Can you work these out from the model? Positions are in its coordinate system, mm. A direction names the side the tool comes from. Give positions to 0.01 mm unless a question says otherwise; leave off trailing zeros. Order: outer loops, then holes, each group sorted by start corner. A loop starts at its lowest first (then second) coordinate and runs counter-clockwise, first axis right, second up. Notation, with made-up numbers: M -16.5,6.25 L 29.5,6.25 A38 cw 29.5,44.25 Z; hole C -35.75,-7.75 d8. An arc over 180 degrees is marked long. One line per question, with ' | ' between items. Start each with the question number.
1) I'm going to push flat-ended pins straight in: pin 1 Ø1.3 at (y, z) = (-0.5, 2) entering from +X; pin 2 Ø1.5 at (x, z) = (0.5, 3.5) entering from +Y; pin 3 Ø1 at (y, z) = (0.5, 2) entering from -X. Where does each tip first touch, or does it pass through?
2) If we section it at C-C, the plane y = 0: Please give me the cut outline in (x, z) (3 decimals).
3) Please list where these lines run through material, in increasing order: line 1 along Y through (x, z) = (0, 1.3); line 2 along Y through (x, z) = (0, 3.2); line 3 along Z through (x, y) = (2.2, -1.45). Write a range as [from, to].
4) If we section it at A-A, the plane z = 1: Please give me the cut outline in (x, y).
5) If we section it at B-B, the plane z = -3: Please give me the cut outline in (x, y).
6) Thinking about a two-plate mould opening in Z: for faces 4 (the flat face through (0, -2.5, -0.5)), 5 (the flat face through (0.25, 0.7, 2.6)), 6 (the flat face through (0.23, 2.64, 0)), which applies, +Z half, -Z half, draft (parallel to the pull), parting line (faces both ways), or undercut?
7) If we section it at D-D, the plane x = -1.1: Please give me the cut outline in (y, z) (3 decimals).
8) For faces 1 (the flat face through (0, 0, 0)), 2 (the cylindrical face through (-0.54, -2.44, 2.51)), 3 (the cylindrical face through (-0.106, 2.923, -0.493)), which set-ups out of +Z, -Z, +X, -X, +Y, -Y let a thin tool reach every point of the face, with its end or its side?
```python
from build123d import *

# Parameters (mm, degrees)
SKETCH1_R           = 2.5
SKETCH1_R_2         = 2
BOSS_EXTRUDE1_DEPTH = 5.1
REVOLVE1_ANGLE      = 180
SKETCH5_R           = 2.925
BOSS_EXTRUDE2_DEPTH = 1
BOSS_EXTRUDE3_DEPTH = 0.25
SKETCH13_W          = 0.5
SKETCH13_H          = 0.5
BOSS_EXTRUDE4_DEPTH = 5
CUT_EXTRUDE2_DEPTH  = 5


with BuildPart() as part:
    # Sketch1 → Boss-Extrude1 (new body)
    with BuildSketch(Plane.XY):
        Circle(SKETCH1_R)
        Circle(SKETCH1_R_2, mode=Mode.SUBTRACT)
    extrude(amount=BOSS_EXTRUDE1_DEPTH)

    # Sketch4 → Revolve1 (revolve)
    with BuildSketch(Plane.XY.offset(5.1)):
        with BuildLine():
            Line((-2, 0), (-2.5, 0))
            ThreePointArc((-2.5, 0), (0, 2.5), (2.5, 0))
            Line((2.5, 0), (2, 0))
            ThreePointArc((2, 0), (0, 2), (-2, 0))
        make_face()
    revolve(axis=Axis((-2.5, 0, 5.1), (1, 0, 0)), revolution_arc=REVOLVE1_ANGLE)

    # Sketch5 → Boss-Extrude2 (add)
    with BuildSketch(Plane(origin=(0, 0, 0), x_dir=(-1, 0, 0), z_dir=(0, 0, -1))):
        Circle(SKETCH5_R)
    extrude(amount=BOSS_EXTRUDE2_DEPTH)

    # Sketch8 → Boss-Extrude3 (add, symmetric)
    with BuildSketch(Plane(origin=(0, 0, 0), x_dir=(0, 0, -1), z_dir=(1, 0, 0))):
        Polygon((0, 1.072701591), (-3.556166294, 1.072701591), (-3.556166294, -0.218813925), (-2.37503672, 0.509733289), (-2.37503672, 0.763620955), (0, 0.763620955), align=None)
        Polygon((-3.556166294, -0.41750862), (-3.330966178, -0.41750862), (-3.330966178, -0.31503842), (-2.37503672, 0.3), (-2.37503672, -0.41750862), (0, -0.41750862), (0, -0.914245357), (-3.556166294, -0.914245357), align=None)
    extrude(amount=BOSS_EXTRUDE3_DEPTH, both=True)

    # Sketch13 → Boss-Extrude4 (add)
    with BuildSketch(Plane(origin=(0, 0, -1), x_dir=(-1, 0, 0), z_dir=(0, 0, -1))):
        with Locations((0.093693205, -1.27)):
            Rectangle(SKETCH13_W, SKETCH13_H)
        with Locations((0.093693205, 1.27)):
            Rectangle(SKETCH13_W, SKETCH13_H)
    extrude(amount=BOSS_EXTRUDE4_DEPTH)

    # Sketch14 → Cut-Extrude2 (cut)
    with BuildSketch(Plane.XY):
        with BuildLine():
            Line((1.518428464, -2.5), (-1.518428464, -2.5))
            ThreePointArc((-1.518428464, -2.5), (0, -2.925), (1.518428464, -2.5))
        make_face()
    extrude(amount=-CUT_EXTRUDE2_DEPTH, mode=Mode.SUBTRACT)


solid = part.part
```
Results found:
1) pin 1: stops at x = 2.5 | pin 2: stops at y = 2.5 | pin 3: stops at x = -2.5
2) outline: M -2.925,-1 L 2.925,-1 L 2.925,0 L 2.5,0 L 2.5,5.1 A2.5 ccw -2.5,5.1 L -2.5,0 L -2.925,0 Z; M -0.25,2.375 L 0.25,2.375 L 0.25,2.841 L -0.25,2.841 Z; M -0.25,3.201 L 0.25,3.201 L 0.25,3.556 L -0.25,3.556 Z; hole M -2,0 L 2,0 L 2,5.1 A2 ccw -2,5.1 Z
3) line 1: y = [-2.5, -2], [-0.91, -0.42], [0.76, 1.07], [2, 2.5] | line 2: y = [-2.5, -2], [-0.91, -0.23], [0, 1.07], [2, 2.5] | line 3: z = [-1, 0]
4) outline: C 0,0 d5; M -0.25,-0.91 L 0.25,-0.91 L 0.25,-0.42 L -0.25,-0.42 Z; M -0.25,0.76 L 0.25,0.76 L 0.25,1.07 L -0.25,1.07 Z; hole C 0,0 d4
5) outline: M -0.34,-1.52 L 0.16,-1.52 L 0.16,-1.02 L -0.34,-1.02 Z; M -0.34,1.02 L 0.16,1.02 L 0.16,1.52 L -0.34,1.52 Z
6) face 4: draft | face 5: undercut | face 6: +Z half
7) outline: M -2.5,-1 L 2.71,-1 L 2.71,0 L 2.245,0 L 2.245,5.1 A2.245 ccw -2.245,5.1 L -2.245,0 L -2.5,0 Z; hole M -1.67,0 L 1.67,0 L 1.67,5.1 A1.67 ccw -1.67,5.1 Z
8) face 1: none | face 2: +Z | face 3: +Z, -Z
